Input: part model. Units: mm. Frame: model coordinates. Coordinates: 2 decimals unless noted, no trailing zeros. Loops run counter-clockwise (first coordinate to the right, second up) from the corner with the lowest first, then second, coordinate; pieces in that order, holes last. Notation, with made-up numbers: M 24.5,-33.5 L 44.5,-33.5 A13 cw 44.5,-29.5 Z; hole C 15,1.5 d8. An arc over 180 degrees is marked long. Use a Markdown table: item, result. Add a question column.
1. Section A-A on y = 49.5. Output: boundary loops of the cut face in (x, z), then the cut area to 3 significant figures.
2. Section D-D on x = -113.5. Output: boundary loops of the cut face in (y, z).
3. Section B-B on y = 21. Output: boundary loops of the cut face in (x, z).
4. Pin query (flat end, axial travel): pin 1 (8 mm diameter, centred on y = 68, z = 38.5, fed in from +X); pin 2 (8 mm diameter, centred on y = 71, z = 32, fed in from -X); pin 3 (3 mm diameter, centred on y = 128, z = 1.5, fed in from -X). Return the tip coordinate at first contact, or that it passes through.
5. Section C-C on z = 46. Output: boundary loops of the cut face in (x, y), then the cut area to 3 significant figures.
6. Line query: L1, parallel to X at y = 49, z = 11.5; L2, parallel to X at y = 106, z = 49; L3, parallel to Y at x = 29.5, z = 20. Output: solid intervals per line, ascending. Write a range as [from, to].
```python
from build123d import *

# Parameters (mm, degrees)
F1_ANGLE      = 30
F2_R          = 3.81
F3_DEPTH      = 138.431
F3_DEPTH_BACK = 138.431
F5_DEPTH      = 2.54


with BuildPart() as f1:
    # F0 (on Top) → F1 (revolve)
    with BuildSketch(Plane.XY):
        with BuildLine():
            Line((-138.43, 0), (-133.35, 0))
            ThreePointArc((-133.35, 0), (0, 133.35), (133.35, 0))
            Line((133.35, 0), (138.43, 0))
            ThreePointArc((138.43, 0), (0, 138.43), (-138.43, 0))
        make_face()
    revolve(axis=Axis((-66.675, 0, 0), (1, 0, 0)), revolution_arc=F1_ANGLE)

    # F2 (on Right) → F3 (cut, two sides)
    with BuildSketch(Plane.YZ) as f3_sk:
        Circle(F2_R)
    extrude(amount=-F3_DEPTH, mode=Mode.SUBTRACT)
    extrude(f3_sk.sketch, amount=F3_DEPTH_BACK, mode=Mode.SUBTRACT)

    # F4 (on Top) → F5 (join)
    with BuildSketch(Plane.XY):
        with BuildLine():
            ThreePointArc((2.54, 133.3258073293), (0, 133.35), (-2.54, 133.3258073293))
            Line((-2.54, 133.3258073293), (-2.54, 125.7058073293))
            Line((-2.54, 125.7058073293), (2.54, 125.7058073293))
            Line((2.54, 125.7058073293), (2.54, 133.3258073293))
        make_face()
    extrude(amount=F5_DEPTH)


solid = f1.part
```
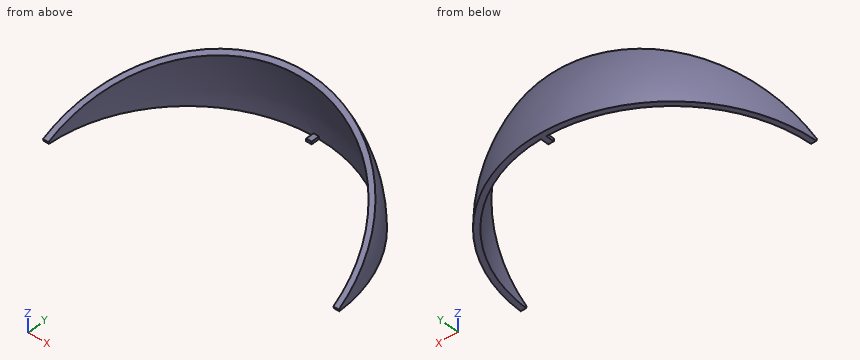
Answers below:
| question | item | result |
|---|---|---|
| 1 | outline | M -129.28,0 L -123.82,0 A123.82 cw -120.48,28.58 L -126.08,28.58 A129.28 ccw Z; M 120.48,28.58 A123.82 cw 123.82,0 L 129.28,0 A129.28 ccw 126.08,28.58 Z |
| 1 | area | 315 mm² |
| 2 | outline | M 60.62,35 A70 cw 70,0 L 79.25,0 A79.25 ccw 68.63,39.63 Z |
| 3 | outline | M -136.83,0 L -131.69,0 A131.69 cw -131.13,12.12 L -136.29,12.12 A136.83 ccw Z; M 131.13,12.12 A131.69 cw 131.69,0 L 136.83,0 A136.83 ccw 136.29,12.12 Z |
| 4 | pin 1 | stops at x = 116.9 |
| 4 | pin 2 | stops at x = -117.07 |
| 4 | pin 3 | stops at x = -56.2 |
| 5 | outline | M -103.44,79.67 L -96.53,79.67 A125.16 cw 96.53,79.67 L 103.44,79.67 A130.56 ccw Z |
| 5 | area | 1,240 mm² |
| 6 | L1 | x = [-128.96, -123.49], [123.49, 128.96] |
| 6 | L2 | x = [-74.34, -64.38], [64.38, 74.34] |
| 6 | L3 | y = [128.5, 133.76] |
